Input: part model. Units: mm. Frame: model coordinates. Face numbers are marked on the shaded views. A direction names the side the tool comes from. Give positions to 0.01 mm unless a question says otherwise; leave off trailing zeros. Loops run counter-clockwise (first coordinate to the right, second up) from the corner with the lowest first, then second, coordinate; pieces in that order, holes last. Notation, with made-up numbers: (47.25, 33) -> (73.25, 33) arc R20 ccw to (73.25, 55) -> close; hole circle Ø10 at (-22, -20.5). An arc over 180 degrees is marked (long way). One line per question, with ' | ' between items.
from build123d import *

# Parameters (mm, degrees)
SKETCH1_W               = 74
SKETCH1_H               = 80
SKETCH1_R               = 30
BOSS_EXTRUDE1_DEPTH     = 6
SKETCH2_R               = 30
SKETCH2_R_2             = 20
BOSS_EXTRUDE2_DEPTH     = 2
SKETCH3_R               = 2.5
CUT_EXTRUDE1_DEPTH      = 2
CHAMFER1_SIZE           = 20
SKETCH4_R               = 2
CUT_EXTRUDE2_DEPTH      = 10
MIRROR2_COPY_1_SKETCH_R = 2
MIRROR2_COPY_1_DEPTH    = 10
CHAMFER2_SIZE           = 1
SKETCH7_W               = 1.90476799
SKETCH7_H               = 4.426812408
CUT_EXTRUDE3_DEPTH      = 1
CUT_EXTRUDE4_DEPTH      = 7


with BuildPart() as part:
    # Sketch1 → Boss-Extrude1 (new body)
    with BuildSketch(Plane.XY):
        with Locations((37, 40)):
            Rectangle(SKETCH1_W, SKETCH1_H)
        with Locations((37, 40)):
            Circle(SKETCH1_R, mode=Mode.SUBTRACT)
    extrude(amount=BOSS_EXTRUDE1_DEPTH)

    # Sketch2 → Boss-Extrude2 (add)
    with BuildSketch(Plane.XY.offset(6)):
        with Locations((37, 40)):
            Circle(SKETCH2_R)
        with Locations((37, 40)):
            Circle(SKETCH2_R_2, mode=Mode.SUBTRACT)
    extrude(amount=-BOSS_EXTRUDE2_DEPTH)

    # Sketch3 → Cut-Extrude1 (cut)
    with BuildSketch(Plane(origin=(0, 0, 4), x_dir=(-1, 0, 0), z_dir=(0, 0, -1))):
        with Locations((-37, 65)):
            Circle(SKETCH3_R)
        with Locations((-15.349364905, 52.5)):
            Circle(SKETCH3_R)
        with Locations((-15.349364905, 27.5)):
            Circle(SKETCH3_R)
        with Locations((-37, 15)):
            Circle(SKETCH3_R)
        with Locations((-58.650635095, 27.5)):
            Circle(SKETCH3_R)
        with Locations((-58.650635095, 52.5)):
            Circle(SKETCH3_R)
    extrude(amount=-CUT_EXTRUDE1_DEPTH, mode=Mode.SUBTRACT)

    # Chamfer1
    chamfer1_edges = [part.edges().sort_by_distance(p)[0] for p in [
        (0, 80, 3),
        (74, 80, 3),
        (74, 0, 3),
        (0, 0, 3),
    ]]
    chamfer(chamfer1_edges, length=CHAMFER1_SIZE)

    # Sketch4 → Cut-Extrude2 (cut)
    with BuildSketch(Plane(origin=(-30, 30, 0), x_dir=(0, 0, 1), z_dir=(-0.707106781, 0.707106781, 0))):
        with Locations((3, 60.568542495)):
            Circle(SKETCH4_R)
        with Locations((3, 52.568542495)):
            Circle(SKETCH4_R)
    cut_extrude2 = extrude(amount=-CUT_EXTRUDE2_DEPTH, mode=Mode.SUBTRACT)

    # Mirror1: Cut-Extrude2 across plane
    add(cut_extrude2.mirror(Plane.ZY.offset(-37)), mode=Mode.SUBTRACT)

    # Mirror2: Cut-Extrude2 across plane
    add(cut_extrude2.mirror(Plane(origin=(0, 40, 0), x_dir=(0, 0, 1), z_dir=(0, -1, 0))), mode=Mode.SUBTRACT)

    # Mirror2 copy 1 sketch → Mirror2 copy 1 (cut)
    with BuildSketch(Plane(origin=(104, 50, 0), x_dir=(0, 0, 1), z_dir=(0.707106781, -0.707106781, 0))):
        with Locations((3, 60.568542495)):
            Circle(MIRROR2_COPY_1_SKETCH_R)
        with Locations((3, 52.568542495)):
            Circle(MIRROR2_COPY_1_SKETCH_R)
    extrude(amount=-MIRROR2_COPY_1_DEPTH, mode=Mode.SUBTRACT)

    # Chamfer2
    chamfer2_edges = [part.edges().sort_by_distance(p)[0] for p in [
        (7, 40, 0),
    ]]
    chamfer(chamfer2_edges, length=CHAMFER2_SIZE)

    # Sketch7 → Cut-Extrude3 (cut)
    with BuildSketch(Plane(origin=(0, 0, 0), x_dir=(-1, 0, 0), z_dir=(0, 0, -1))):
        with Locations((-37, 77.786593796)):
            Rectangle(SKETCH7_W, SKETCH7_H)
    extrude(amount=-CUT_EXTRUDE3_DEPTH, mode=Mode.SUBTRACT)

    # Sketch8 → Cut-Extrude4 (cut, through all)
    with BuildSketch(Plane.XY.offset(6)):
        Polygon((0, 60), (7.071067812, 60), (20, 72.928932188), (20, 80), align=None)
        Polygon((54, 80), (54, 72.928932188), (66.928932188, 60), (74, 60), align=None)
        Polygon((66.928932188, 20), (74, 20), (54, 0), (54, 7.071067812), align=None)
        Polygon((0, 20), (7.071067812, 20), (20, 7.071067812), (20, 0), align=None)
    extrude(amount=-CUT_EXTRUDE4_DEPTH, mode=Mode.SUBTRACT)


solid = part.part
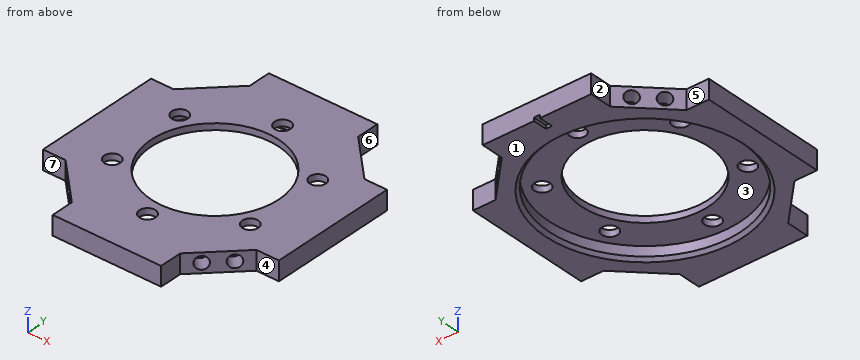
1. Section query A-A (y = 40). Output: boundary loops of the cut face in (x, z), then the cut area to 3 significant figures.
Determined:
outline: (0, 0) -> (6, 0) -> (7, 1) -> (7, 4) -> (17, 4) -> (17, 6) -> (0, 6) -> close; (57, 4) -> (67, 4) -> (67, 1) -> (68, 0) -> (74, 0) -> (74, 6) -> (57, 6) -> close | area: 123 mm2
2. Section query B-B (y = 27.5). Count the separate pieces of the cut face and the enclosed holes in it, then the cut area to 3 significant figures.
Determined:
separate pieces: 4 | enclosed holes: 0 | area: 142 mm2
3. Pull-direction query (X, two-part tool) for the marked faces 1, 2 and 3; classes: pulls with the +X half, pulls with the -X half, needs draft (parallel to the pull), parting line crosses it, or undercut.
Determined:
face 1: needs draft | face 2: pulls with the -X half | face 3: undercut
4. Pin query (flat end, axial travel): P1, Ø4.5, axis at x = 58.65, y = 52.5, coming from the +Z side; P2, Ø3, axis at y = 76.5, z = 3, coming from the +X side; P3, Ø2, axis at x = 33.5, y = 62, coming from the -Z side; P4, Ø1, axis at x = 61, z = 5, coming from the +Y side. Return the tip coordinate at first contact, or that it passes through.
Determined:
P1: passes through | P2: stops at x = 54 | P3: stops at z = 4 | P4: stops at y = 66.43
5. Ray query, line 1 along Y through (x, z) = (37, 4.4); line 2 along Y through (x, z) = (25, 2.5); line 3 along Y through (x, z) = (61.5, 4.5). Return the intervals inside material, ascending. Write a range as from..to.
Determined:
line 1: y = 0..12.5, 17.5..20, 60..62.5, 67.5..80 | line 2: y = 0..12.5, 67.5..80 | line 3: y = 14.57..16.29, 20.03..59.97, 63.71..65.43
6. Reachability of the marked faces 4, 5, 6 and 7 from +Z, -Z, +X, -X, +Y, -Y: full face, straight path, thin tool, end or side. Return the list, or none.
Determined:
face 4: +Z, -Z, +X, -Y | face 5: +Z, -Z, -X, +Y | face 6: +Z, -Z, +X, +Y | face 7: +Z, -Z, -X, -Y
